Build history of the part. All positions in model axes, mm. Face numbers are marked on the shaded views. Coordinates: 2 decimals unless noted, no trailing zeros. Loops run counter-clockwise (first coordinate to the right, second up) from the corner with the lowest first, then second, coordinate; pieces in that order, holes last.
Item 1: Drill centre lines: line 1 along Y through (x, z) = (1788, 2.75); line 2 along Y through (x, z) = (613.31, 4.25); line 3 along Y through (x, z) = (1839, 74). Where is each one in solid material? Low to high.
Item 2: Mould opens along Y. For the marked faces 1 and 2 say: released by +Y, released by -Y, zero draft, split by the parting line, or undercut.
Item 3: Cut at C-C (y = -384.5). List the corners of the cut face in (x, z).
Item 4: Cut at D-D (x = 1952.5). List the corners of the cut face in (y, z).
Item 5: Cut at A-A (x = 553). List the corners of the cut face in (y, z).
Item 6: Flat gauge pins, fed straight in: pin 1 (1.5 mm diameter, centred on x = 1311.5, z = 124, fed in from +Y); pin 2 (5 mm diameter, centred on x = 788.5, z = 123, fed in from -Y); pin 3 (19.5 mm diameter, centred on x = 849, y = -739.5, fed in from +Z). Where does each tip first touch, or does it go through?
Item 7: Cut at B-B (z = 130). List the corners of the cut face in (x, y).
from build123d import *

# Parameters (mm, degrees)
F1_DEPTH       = 1985
F3_DEPTH       = 710
F5_DEPTH       = 1575
F7_DEPTH       = 10
F9_DEPTH       = 140
F10_R          = 10
F11_DEPTH      = 25
F12_R          = 20
F13_DEPTH      = 15
F14_R          = 20
F15_DEPTH      = 25
F17_DEPTH      = 177
F17_DEPTH_BACK = 25


with BuildPart() as f1:
    # F0 (on Right) → F1 (new body)
    with BuildSketch(Plane.YZ):
        Polygon((0, 10), (0, 0), (10, 0), (75, 0), (75, 10), (10, 10), (10, 150), (0, 150), align=None)
    extrude(amount=F1_DEPTH)

    # F2 (on face) → F3 (join)
    with BuildSketch(Plane.XZ):
        Polygon((1910, 10), (1910, 0), (1920, 0), (1985, 0), (1985, 10), (1920, 10), (1920, 150), (1910, 150), align=None)
    extrude(amount=F3_DEPTH)



with BuildPart() as f5:
    # F4 (on face) → F5 (new body)
    with BuildSketch(Plane.YZ.offset(1985)):
        Polygon((-720, 150), (-720, 10), (-785, 10), (-785, 0), (-720, 0), (-710, 0), (-710, 10), (-710, 150), align=None)
    extrude(amount=-F5_DEPTH)


with BuildPart() as f7:
    # F6 (on Top) → F7 (new body)
    with BuildSketch(Plane.XY):
        Polygon((485, -710), (75, 0), (0, 0), (410, -710), align=None)
    extrude(amount=F7_DEPTH)


with BuildPart() as f1_1:
    add(f1.part)

    add(f5.part)  # F9 merges F5

    add(f7.part)  # F9 merges F7
    # F8 (on face) → F9 (join)
    with BuildSketch(Plane.XY.offset(10)):
        Polygon((485, -710), (75, 0), (65, 0), (475, -710), align=None)
    extrude(amount=F9_DEPTH)

    # F10 (on face) → F11 (cut)
    with BuildSketch(Plane.XY.offset(10)):
        with Locations((613.31, -752.5)):
            Circle(F10_R)
        with Locations((1413.31, -752.5)):
            Circle(F10_R)
        with Locations((1788, 42.5)):
            Circle(F10_R)
        with Locations((188, 42.5)):
            Circle(F10_R)
    extrude(amount=-F11_DEPTH, mode=Mode.SUBTRACT)

    # F12 (on face) → F13 (cut)
    with BuildSketch(Plane.XZ.offset(720)):
        with Locations((442.5, 80)):
            Circle(F12_R)
        with Locations((1950, 80)):
            Circle(F12_R)
    extrude(amount=-F13_DEPTH, mode=Mode.SUBTRACT)

    # F14 (on face) → F15 (cut)
    with BuildSketch(Plane(origin=(0, 10, 0), x_dir=(-1, 0, 0), z_dir=(0, 1, 0))):
        with Locations((-1952.5, 80)):
            Circle(F14_R)
        with Locations((-32.5, 80)):
            Circle(F14_R)
    extrude(amount=-F15_DEPTH, mode=Mode.SUBTRACT)

    # F16 (on face) → F17 (cut, two sides)
    with BuildSketch(Plane.XY.offset(10)) as f17_sk:
        Polygon((453.309859, -785), (410, -710), (410, -785), align=None)
    extrude(amount=F17_DEPTH, mode=Mode.SUBTRACT)
    extrude(f17_sk.sketch, amount=-F17_DEPTH_BACK, mode=Mode.SUBTRACT)


solid = f1_1.part
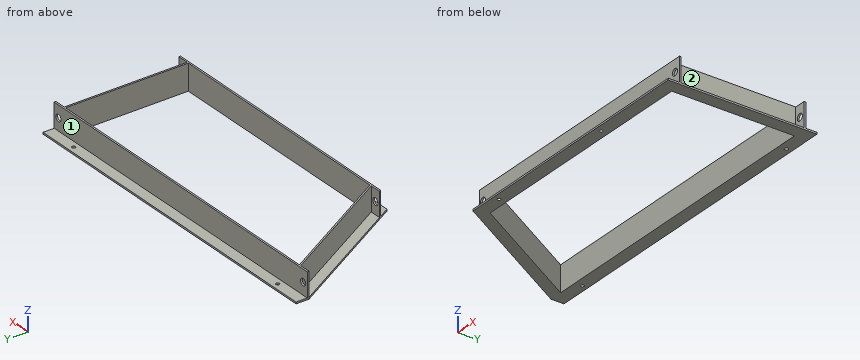
Filled sheet:
1. line 1: y = -785 to -710, 0 to 32.5, 52.5 to 75
1. line 2: y = -785 to -762.5, -742.5 to -710, 0 to 75
1. line 3: y = -720 to -710, 0 to 10
2. face 1: released by +Y
2. face 2: undercut
3. outline: (222.04, 0) - (297.04, 0) - (297.04, 150) - (287.04, 150) - (287.04, 10) - (222.04, 10) - close; (1910, 0) - (1985, 0) - (1985, 10) - (1920, 10) - (1920, 150) - (1910, 150) - close
4. outline: (-785, 0) - (75, 0) - (75, 10) - (10, 10) - (10, 60) - (0, 60) - (0, 10) - (-710, 10) - (-710, 60.16) - (-720, 60.16) - (-720, 10) - (-785, 10) - close; (-720, 99.84) - (-710, 99.84) - (-710, 150) - (-720, 150) - close; (0, 100) - (10, 100) - (10, 150) - (0, 150) - close
5. outline: (-785, 0) - (-710, 0) - (-710, 150) - (-720, 150) - (-720, 10) - (-785, 10) - close; (0, 0) - (75, 0) - (75, 10) - (10, 10) - (10, 150) - (0, 150) - close
6. pin 1: stops at y = 10
6. pin 2: stops at y = -720
6. pin 3: stops at z = 10
7. outline: (0, 0) - (65, 0) - (475, -710) - (410, -710) - (415.77, -720) - (1985, -720) - (1985, -710) - (1920, -710) - (1920, 0) - (1985, 0) - (1985, 10) - (0, 10) - close; hole (75, 0) - (485, -710) - (1910, -710) - (1910, 0) - close
